Autodesk Inventor part; units mm, degrees
ref_plane "Work Plane1" through (14.1718, 0, 0) normal (0, 0.7071, -0.7071) x (-1, 0, 0)
ref_plane "YZ Plane" through (0, 0, 0) normal (1, 0, 0) x (0, 1, 0)
ref_plane "XZ Plane" through (0, 0, 0) normal (0, 1, 0) x (-1, 0, 0)
sketch "Skizze1" plane through (0, 0, 0) normal (1, 0, 0) x (0, 1, 0)
  line L0 (0, -4.9497) -> (-4.9497, 0)
  line L1 (-4.9497, 0) -> (0, 4.9497)
  line L2 (0, 4.9497) -> (4.9497, 0)
  line L3 (4.9497, 0) -> (0, -4.9497)
  line L4 (-6.9296, 0) -> (6.9296, 0)
  point P0 (0, 0)
  point P1 (0, 0)
  dimension "d0" = 9.8995
extrude "Körper" add sketch "Skizze1" along normal blind 2.2
sketch "Skizze2" plane through (0, 0, 0) normal (-1, 0, 0) x (0, 0, 1)
  point P0 (0, 0)
  point P1 (0, 0)
hole "Gewinde" at (0, 0, 0) direction (1, 0, 0) diameter 3.242 end through all
chamfer "Fase1" distance 0.3789 angle 30 1 edges at (0, 0, -1.621) measured on face at (0, -2.0082, 2.0544)
chamfer "Fase2" distance 0.3789 angle 30 1 edges at (2.2, 0, -1.621) measured on face at (2.2, -2.0082, 2.0544)
ref_plane "Work Plane1" through (14.1718, 0, 0) normal (0, 0.7071, -0.7071) x (-1, 0, 0)
equation "\"d0\" = 1.41421 * SW"
equation "\"d1\" = KOH"
equation "\"d3\" = -0.5 * GD1 + 0.5 * NND"
equation "\"d35\" = -0.5 * GD1 + 0.5 * NND"
equation "\"d5\" = -0.5 * GD1 + 0.5 * NND"
equation "\"d36\" = -0.5 * GD1 + 0.5 * NND"
equation "\"NND\" = 4"
equation "\"KOH\" = 2.2"
equation "\"SW\" = 7"
equation "\"GUL\" = 0.541266 * PTC"
equation "\"THREADDIA\" = 4"
equation "\"TOA\" = 30deg"
equation "\"PTC\" = 0.7"
equation "\"E0\" = 8.9"
equation "\"GAL\" = 0.541266 * PTC"
properties part number "DIN 562 - M4" material "Stahl, weich"
Can you work these out from the model? Positions are in its coordinate system, mm. Give positions to 0.01 mm unless a question says otherwise; leave off trailing zeros. Loops run counter-clockwise (first coordinate to the right, second up) from the corner with the lowest first, then second, coordinate; pieces in that order, holes last. Notation, with made-up numbers: M -40,21.5 L 14,21.5 A19 cw 14,42.5 Z; hole C -24.75,89 d1. An arc over 180 degrees is marked long. One line per item, written item: value.
1) Imagine slicing it at A-A on x = 0.75. Write out the boundary of the cut face in (y, z), and give its area (3 significant figures).
Geometry check:
outline: M -4.95,0 L 0,-4.95 L 4.95,0 L 0,4.95 Z; hole C 0,0 d3.24
area: 40.7 mm²
2) Imagine slicing it at C-C on y = 2.5. Write out the boundary of the cut face in (x, z).
Geometry check:
outline: M 0,-2.45 L 2.2,-2.45 L 2.2,2.45 L 0,2.45 Z
3) Imagine slicing it at B-B on z = 3.5. Write out the boundary of the cut face in (x, y).
Geometry check:
outline: M 0,-1.45 L 2.2,-1.45 L 2.2,1.45 L 0,1.45 Z
4) I'm going to push flat-ended pins straight in: pin 1 (1.5 mm diameter, centred on y = 0, z = 4, fed in from -X); pin 2 (2.5 mm diameter, centred on y = 0, z = 0, fed in from +X). Where does each tip first touch, or does it pass through?
Geometry check:
pin 1: stops at x = 0
pin 2: passes through
5) Thinking about a two-plate mould opening in Z: for faces 1 (the face through (1.08, -2.51, 2.44)), 2 (the face through (2.2, -0.1, 2.3)), 3 (the face through (1.112, 1.438, 0.748)), 4 (the face through (1.08, -2.44, -2.51)), which applies, +Z half, -Z half, draft (parallel to the pull), parting line (faces both ways), or undercut?
Geometry check:
face 1: +Z half
face 2: draft
face 3: undercut
face 4: -Z half
6) Please list where these lines run through material, in increasing order: line 1 (Z direction, x = 1.55, y = 2.75); line 2 (Z direction, x = 1, y = 1.25); line 3 (X direction, y = 1.75, z = 0.5).
Geometry check:
line 1: z = -2.2 to 2.2
line 2: z = -3.7 to -1.03, 1.03 to 3.7
line 3: x = 0.1 to 2.1
